from build123d import *

# Parameters (mm, degrees)
F0_W     = 4.6872794628
F0_H     = 85.9219655395
F1_DEPTH = 6.35
F2_W     = 4.8930570483
F2_H     = 85.9219655395
F2_W_2   = 70.9142880514
F2_H_2   = 5.7498048991
F3_DEPTH = 6.35
F4_R     = 5.08
F5_SIZE  = 2.54
F6_R     = 5.5162343309
F6_R_2   = 1.8756395143
F7_DEPTH = 2.54
F8_DEPTH = 3.048


with BuildPart() as f1:
    # F0 (on Front) → F1 (new body, symmetric)
    with BuildSketch(Plane.XZ):
        Polygon((76.0237202048, -5.7498048991), (76.0237202048, 0), (71.336440742, 0), (-71.336440742, 0), (-76.0237202048, 0), (-76.0237202048, -5.7498048991), (0, -5.7498048991), align=None)
        with Locations((-73.6800804734, 42.9609827697)):
            Rectangle(F0_W, F0_H)
        with Locations((73.6800804734, 42.9609827697)):
            Rectangle(F0_W, F0_H)
    extrude(amount=F1_DEPTH, both=True)

    # F2 (on Right) → F3 (join, symmetric)
    with BuildSketch(Plane.YZ):
        with Locations((79.7009654343, 42.9609827697)):
            Rectangle(F2_W, F2_H)
        with Locations((41.7972928844, -2.8749024495)):
            Rectangle(F2_W_2, F2_H_2)
        Polygon((82.1474939585, 0), (77.2544369102, 0), (77.2544369102, -5.7498048991), (82.3985040188, -5.7498048991), align=None)
    extrude(amount=F3_DEPTH, both=True)

    # F4
    f4_edges = [f1.edges().sort_by_distance(p)[0] for p in [
        (0, 77.254437, 0),
        (-71.336441, 0, 0),
        (71.336441, 0, 0),
        (-76.02372, 0, -5.749805),
        (76.02372, 0, -5.749805),
        (0, 82.398504, -5.749805),
    ]]
    fillet(f4_edges, radius=F4_R)

    # F5
    f5_edges = [f1.edges().sort_by_distance(p)[0] for p in [
        (-73.68008, -6.35, 85.921966),
        (-73.68008, 6.35, 85.921966),
        (73.68008, -6.35, 85.921966),
        (73.68008, 6.35, 85.921966),
        (6.35, 79.700965, 85.921966),
        (-6.35, 79.700965, 85.921966),
    ]]
    chamfer(f5_edges, length=F5_SIZE)

    # F6 (on face) → F7 (join)
    with BuildSketch(Plane.XY):
        Circle(F6_R)
        Circle(F6_R_2, mode=Mode.SUBTRACT)
    extrude(amount=F7_DEPTH)

    # F8 (add): a face of the model
    f8_faces = [f1.faces().sort_by_distance(p)[0] for p in [
        (0, 0, 0),
    ]]
    extrude(f8_faces, amount=F8_DEPTH)


solid = f1.part
Build history of the part. All positions in model axes, mm. A direction names the side the tool comes from. Coordinates: 2 decimals unless noted, no trailing zeros. Order: outer loops, then holes, each group sorted by start corner. A loop starts at its lowest first (then second) coordinate and runs counter-clockwise, first axis right, second up. Notation, with made-up numbers: (75.25, 66.5) - (123.25, 66.5) arc R18 cw to (123.25, 70.5) - close; hole circle Ø1 at (-1.75, -6). An arc over 180 degrees is marked (long way). Write each question's results on one line, items separated by ' | '. Start each with the question number.
Item 1: Flat gauge pins, fed straight in: pin 1 (1.9 mm diameter, centred on x = -1, y = 0.5, fed in from +Z); pin 2 (4 mm diameter, centred on x = 0, z = 56, fed in from -Y); pin 3 (10 mm diameter, centred on x = 1, z = 48, fed in from +Y); pin 4 (12 mm diameter, centred on y = 57.5, z = 10, fed in from -X). Where does each tip first touch, or does it go through?
Item 2: Band-saw the part on D-D on y = 18. Write the cut outline in (x, z).
Item 3: Wall check: probe 1 along X at (y, z) = (4.5, 69.5); probe 2 along Y at (x, z) = (-5.5, 80.5); probe 3 along X at (y, z) = (77.5, 73). Give the ranges that are in metal, low to high. Write a range as [from, to].
Item 4: Band-saw the part on A-A on z = 61. Write the cut outline in (x, y).
Item 5: Band-saw the part on B-B on x = 0. Write the cut outline in (y, z), and give its area (3 significant figures).
Item 6: Band-saw the part on C-C on y = 0. Write the cut outline in (x, z), and give its area (3 significant figures).
Item 7: Mould opens along X. For faces 4 (the face through (-6.35, 78, 19)), 5 (the face through (0, 80, 85.922)), 6 (the face through (1.79, 0.56, 2.79)) say: released by +X, released by -X, zero draft, split by the parting line, or undercut.
Item 8: Tool access for faces 1 (the face through (0, 12, 0)), 2 (the face through (6.35, 78, 19)), 3 (the face through (71.336, 0, 45)): list every direction of +Z, -Z, +X, -X, +Y, -Y with a clear straight run to the whole face (end or side of a thin tool).
Numbers:
1) pin 1: z = 3.05 | pin 2: y = 77.25 | pin 3: y = 82.15 | pin 4: through
2) outline: (-6.35, -5.75) - (6.35, -5.75) - (6.35, 0) - (-6.35, 0) - close
3) probe 1: [-76.02, -71.34], [71.34, 76.02] | probe 2: [77.25, 82.15] | probe 3: [-6.35, 6.35]
4) outline: (-76.02, -6.35) - (-71.34, -6.35) - (-71.34, 6.35) - (-76.02, 6.35) - close; (-6.35, 77.25) - (6.35, 77.25) - (6.35, 82.15) - (-6.35, 82.15) - close; (71.34, -6.35) - (76.02, -6.35) - (76.02, 6.35) - (71.34, 6.35) - close
5) outline: (-6.35, -5.75) - (77.09, -5.75) arc R5.08 ccw to (82.17, -0.45) - (82.15, 0) - (82.15, 85.92) - (77.25, 85.92) - (77.25, 5.08) arc R5.08 cw to (72.17, 0) - (5.52, 0) - (5.52, 2.54) - (1.88, 2.54) - (1.88, 3.05) - (-1.88, 3.05) - (-1.88, 2.54) - (-5.52, 2.54) - (-5.52, 0) - (-6.35, 0) - close | area: 959 mm^2
6) outline: (-76.02, -0.67) arc R5.08 ccw to (-70.94, -5.75) - (70.94, -5.75) arc R5.08 ccw to (76.02, -0.67) - (76.02, 85.92) - (71.34, 85.92) - (71.34, 5.08) arc R5.08 cw to (66.26, 0) - (5.52, 0) - (5.52, 2.54) - (1.88, 2.54) - (1.88, 3.05) - (-1.88, 3.05) - (-1.88, 2.54) - (-5.52, 2.54) - (-5.52, 0) - (-66.26, 0) arc R5.08 cw to (-71.34, 5.08) - (-71.34, 85.92) - (-76.02, 85.92) - close | area: 1,710 mm^2
7) face 4: released by -X | face 5: zero draft | face 6: undercut
8) face 1: +Z | face 2: +Z, -Z, +X, +Y | face 3: +Z, +Y, -Y
